Design review of the part built by this model. Coordinates are the model's own, in mm. A direction names the side the tool comes from. Coordinates: 2 decimals unless noted, no trailing zeros. Write each loop counter-clockwise with the first axis right and the second up, starting at its lowest first coordinate (ties: lowest second). Pieces come first, ordered by that corner, then holes.
Q1. Take a section at A-A, the plane x = 6. Write out the cut boundary in (y, z), plus the area to 3 significant figures.
Q2. For L1, parallel to X at y = -22.05, z = 8; L2, parallel to Z at x = 20.5, y = -13.5; L3, parallel to Y at x = 18, z = 9.25, list the stretches that pass through material, from the lowest coordinate up.
Q3. Take a section at D-D, the plane z = 8. Write out the cut boundary in (x, y), plus the area to 3 significant figures.
Q4. The part is to be moulded in two halves that separate along X. For faces 6 (the flat face through (-0.348, -22, 2)), 7 (the flat face through (3.8, 6.61, 0.5)), 8 (the cylindrical face through (24.839, -21.883, 10.574)), say which applies: released by +X, released by -X, zero draft, split by the parting line, or undercut.
Q5. For pin 1 Ø1.5 at (x, z) = (17.5, 10) entering from +Y; pin 2 Ø8.5 at (x, y) = (-6.5, -12) entering from +Z; pin 3 Ø4 at (y, z) = (-8.5, 4.5) entering from -X; pin 4 Ø0.5 at (x, y) = (2, -22) entering from -Z, all flat-tipped, find the tip position at first contact; note any pin that passes through.
Q6. Take a section at B-B, the plane z = 2. Write out the cut boundary in (x, y), plus the area to 3 significant figures.
Q7. For faces 1 (the flat face through (4.2, -12.19, 0.5)), 2 (the flat face through (4, -22, 5)), 3 (the flat face through (8.786, -18.4, 0.8)), 4 (the cylindrical face through (-15.38, -21.88, 6.73)), 5 (the flat face through (4, -21.39, 7)), list the 3-axis set-ups (+Z, -Z, +X, -X, +Y, -Y) from which the entire face can be reached by the end or side of a thin tool; tool diameter is ignored.
Q8. Take a section at C-C, the plane x = -1. Write out the cut boundary in (y, z), plus the area to 3 significant figures.
from build123d import *

# Parameters (mm, degrees)
SKETCH1_W           = 44.5
SKETCH1_H           = 29
BOSS_EXTRUDE1_DEPTH = 12
SKETCH2_W           = 11
SKETCH2_H           = 28
CUT_EXTRUDE1_DEPTH  = 52.240207176
SKETCH3_R           = 1.6
SKETCH3_W           = 9.133902139
SKETCH3_H           = 9.2
CUT_EXTRUDE2_DEPTH  = 16.77
SKETCH4_R           = 1.6
CUT_EXTRUDE4_DEPTH  = 16.77
FILLET1_R           = 5
FILLET2_R           = 5
SKETCH11_W          = 9.133756838
SKETCH11_H          = 2
CUT_EXTRUDE7_DEPTH  = 5


with BuildPart() as part:
    # Sketch1 → Boss-Extrude1 (new body)
    with BuildSketch(Plane.XY):
        with Locations((4.092804291, -7.889927007)):
            Rectangle(SKETCH1_W, SKETCH1_H)
    extrude(amount=BOSS_EXTRUDE1_DEPTH)

    # Sketch2 → Cut-Extrude1 (cut, through all)
    with BuildSketch(Plane.ZY.offset(18.157195709)):
        with Locations((6.5, -7.389927007)):
            Rectangle(SKETCH2_W, SKETCH2_H)
    extrude(amount=-CUT_EXTRUDE1_DEPTH, mode=Mode.SUBTRACT)

    # Sketch3 → Cut-Extrude2 (cut)
    with BuildSketch(Plane.XY.offset(1)):
        with Locations((-16.195951252, 4.110072993)):
            Circle(SKETCH3_R)
        with Locations((24.504048748, -12.189927007)):
            Circle(SKETCH3_R)
        with Locations((4.21890888, -16.789927007)):
            Rectangle(SKETCH3_W, SKETCH3_H)
    extrude(amount=-CUT_EXTRUDE2_DEPTH, mode=Mode.SUBTRACT)

    # Sketch4 → Cut-Extrude4 (cut)
    with BuildSketch(Plane(origin=(0, -21.389927007, 0), x_dir=(1, 0, 0), z_dir=(0, 1, 0))):
        with Locations(Location((-14.407195709, -8, 0), (0, 0, 270))):
            Circle(SKETCH4_R)
        with Locations(Location((22.592804291, -8, 0), (0, 0, 270))):
            Circle(SKETCH4_R)
    extrude(amount=-CUT_EXTRUDE4_DEPTH, mode=Mode.SUBTRACT)

    # Fillet1
    fillet1_edges = [part.edges().sort_by_distance(p)[0] for p in [
        (-18.157195709, -21.889927007, 12),
    ]]
    fillet(fillet1_edges, radius=FILLET1_R)

    # Fillet2
    fillet2_edges = [part.edges().sort_by_distance(p)[0] for p in [
        (26.342804291, -21.889927007, 12),
    ]]
    fillet(fillet2_edges, radius=FILLET2_R)

    # Sketch11 → Cut-Extrude7 (cut)
    with BuildSketch(Plane(origin=(0, 0, 0), x_dir=(-1, 0, 0), z_dir=(0, 0, -1))):
        with Locations((-4.21898153, -22.389927007)):
            Rectangle(SKETCH11_W, SKETCH11_H)
    extrude(amount=-CUT_EXTRUDE7_DEPTH, mode=Mode.SUBTRACT)


solid = part.part
Responses:
1. outline: (-22.39, 5) - (-21.39, 5) - (-21.39, 12) - (-22.39, 12) - close; (-12.19, 0) - (6.61, 0) - (6.61, 1) - (-12.19, 1) - close
1. area: 25.8 mm2
2. L1: x = -18.06 to -16.01, -12.81 to 20.99, 24.19 to 26.24
2. L2: z = 0 to 1
2. L3: y = -22.39 to -21.39
3. outline: (-18.06, -22.39) - (-16.01, -22.39) - (-16.01, -21.39) - (-18.06, -21.39) - close; (-12.81, -22.39) - (20.99, -22.39) - (20.99, -21.39) - (-12.81, -21.39) - close; (24.19, -22.39) - (26.24, -22.39) - (26.24, -21.39) - (24.19, -21.39) - close
3. area: 37.9 mm2
4. face 6: undercut
4. face 7: zero draft
4. face 8: released by +X
5. pin 1: stops at y = -21.39
5. pin 2: stops at z = 1
5. pin 3: passes through
5. pin 4: stops at z = 5
6. outline: (-18.16, -22.39) - (-0.35, -22.39) - (-0.35, -21.39) - (-18.16, -21.39) - close; (8.79, -22.39) - (26.34, -22.39) - (26.34, -21.39) - (8.79, -21.39) - close
6. area: 35.4 mm2
7. face 1: +Z, -Z, -Y
7. face 2: -Z, +Y, -Y
7. face 3: -Z, -Y
7. face 4: +Y, -Y
7. face 5: +Z, +X, -X, +Y
8. outline: (-22.39, 0) - (6.61, 0) - (6.61, 1) - (-21.39, 1) - (-21.39, 12) - (-22.39, 12) - close
8. area: 40.0 mm2
